CAD build for the part. Positions are in the model's coordinates, mm. Give positions to 0.01 mm unless a question says otherwise; leave off trailing zeros. Loops run counter-clockwise (first coordinate to the right, second up) from the corner with the lowest first, then second, coordinate; pieces in that order, holes last. Notation, with made-up numbers: M 68,4.5 L 119,4.5 A11 cw 119,10.5 Z; hole C -21,11 d7. An arc over 180 degrees is marked long. One line per question, with ' | ' between items.
```python
from build123d import *

# Parameters (mm, degrees)
BOSS_EXTRUDE1_DEPTH = 3
SKETCH3_R           = 1.5
CUT_EXTRUDE1_DEPTH  = 128.116518704


with BuildPart() as part:
    # Sketch2 → Boss-Extrude1 (new body)
    with BuildSketch(Plane(origin=(0, 0, 0), x_dir=(1, 0, 0), z_dir=(0, 1, 0))):
        with BuildLine():
            Line((0, 0), (75, 0))
            Line((75, 0), (75, 16))
            Line((75, 16), (60.175624146, 26.380139722))
            Line((60.175624146, 26.380139722), (52.5, 31.75466961))
            Line((52.5, 31.75466961), (52.5, 49))
            Line((52.5, 49), (77.774698645, 72.564473175))
            Line((77.774698645, 72.564473175), (79.67816092, 93.959773343))
            ThreePointArc((79.67816092, 93.959773343), (37.5, 99), (-4.67816092, 93.959773343))
            Line((-4.67816092, 93.959773343), (-2.774698645, 72.564473175))
            Line((-2.774698645, 72.564473175), (22.5, 49))
            Line((22.5, 49), (22.5, 31.75466961))
            Line((22.5, 31.75466961), (14.824375854, 26.380139722))
            Line((14.824375854, 26.380139722), (0, 16))
            Line((0, 16), (0, 0))
        make_face()
    extrude(amount=BOSS_EXTRUDE1_DEPTH)

    # Sketch3 → Cut-Extrude1 (cut, through all)
    with BuildSketch(Plane(origin=(0, 3, 0), x_dir=(1, 0, 0), z_dir=(0, 1, 0))):
        with Locations(Location((26.5, 69.377334805, 0), (0, 0, 270))):
            Circle(SKETCH3_R)
        with Locations(Location((48.5, 69.377334805, 0), (0, 0, 90))):
            Circle(SKETCH3_R)
        with Locations(Location((48.5, 11.377334805, 0), (0, 0, 270))):
            Circle(SKETCH3_R)
        with Locations(Location((26.5, 11.377334805, 0), (0, 0, 90))):
            Circle(SKETCH3_R)
    extrude(amount=-CUT_EXTRUDE1_DEPTH, mode=Mode.SUBTRACT)


solid = part.part
```
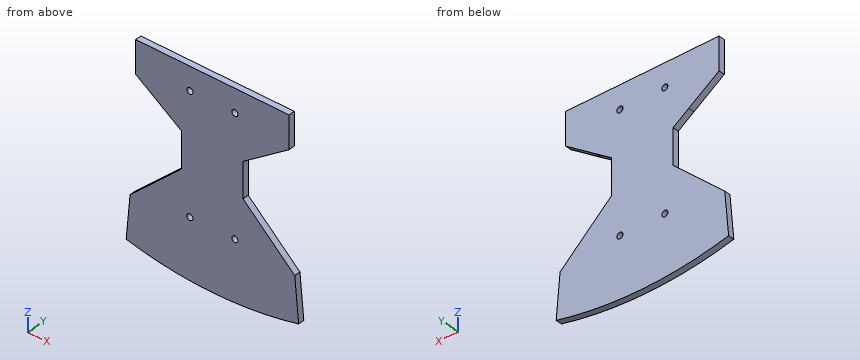
Item 1: Saw through at A-A on y = 0.8. Give the cut face in (x, z).
Conclusion:
outline: M -4.68,-93.96 A179 ccw 79.68,-93.96 L 77.77,-72.56 L 52.5,-49 L 52.5,-31.75 L 75,-16 L 75,0 L 0,0 L 0,-16 L 22.5,-31.75 L 22.5,-49 L -2.77,-72.56 Z; hole C 26.5,-69.38 d3; hole C 26.5,-11.38 d3; hole C 48.5,-69.38 d3; hole C 48.5,-11.38 d3
Item 2: Saw through at C-C on z = -5.5. Give the cut face in (x, y).
Conclusion:
outline: M 0,0 L 75,0 L 75,3 L 0,3 Z
Item 3: Saw through at B-B on x = 48.5. Give the cut face in (y, z).
Conclusion:
outline: M 0,-98.66 L 3,-98.66 L 3,-70.88 L 0,-70.88 Z; M 0,-67.88 L 3,-67.88 L 3,-12.88 L 0,-12.88 Z; M 0,-9.88 L 3,-9.88 L 3,0 L 0,0 Z
Item 4: Saw through at D-D on z = -38. Give the cut face in (x, y).
Conclusion:
outline: M 22.5,0 L 52.5,0 L 52.5,3 L 22.5,3 Z
Item 5: Drill centre lines: line 1 along Z through (x, y) = (53, 2.55); line 2 along X through (y, z) = (2.95, -13); line 3 along Z through (x, y) = (17, 0.25). Where is each one in solid material? Low to high. Write a range as [from, to].
Conclusion:
line 1: [-98.33, -49.47], [-31.4, 0] | line 2: [0, 75] | line 3: [-97.82, -54.13], [-27.9, 0]
Item 6: Drop flat-ended pins along their axis: P1, Ø1.5, axis at y = 1, z = -39.5, coming from the +X side; P2, Ø1.5, axis at y = 1, z = -8, coming from the -X side; P3, Ø1, axis at x = 32.5, y = 1.5, coming from the +Z side. Give the stop position or say it passes through.
Conclusion:
P1: x = 52.5 | P2: x = 0 | P3: z = 0
